Check sheet for the modelled part. Datum: model origin and axes. Units: mm. Face numbers are marked on the shaded views. A direction names the side the tool comes from. Round coordinates to 2 decimals unless told otherwise and drop trailing zeros. Order: outer loops, then holes, each group sorted by start corner. A loop starts at its lowest first (then second) coordinate and runs counter-clockwise, first axis right, second up.
(1) Sectioned sample at C-C, the plane x = 6.5. Enter the section's corners in (y, z).
(2) Sectioned sample at B-B, the plane z = 0. Enter the section's corners in (x, y).
(3) Sectioned sample at A-A, the plane y = -9.5. Enter the section's corners in (x, z), and give its area (3 significant figures).
(4) Sectioned sample at D-D, the plane y = -21. Enter the section's corners in (x, z).
(5) Tool access check on the marked faces 1 and 2. Record the directions out of +Z, -Z, +X, -X, +Y, -Y that give a thin tool (end or side, any length) a straight path to the whole face; none if there is none.
(6) Thickness scan on probe 1 along Z at (x, y) = (9.5, -20.5); probe 2 along X at (y, z) = (-9, -25); probe 3 along Z at (x, y) = (4, -12). Record the ranges inside material, lowest first.
```python
from build123d import *

# Parameters (mm, degrees)
BOSS_EXTRUDE1_DEPTH = 13
BOSS_EXTRUDE4_DEPTH = 2


with BuildPart() as part:
    # Sketch1 → Boss-Extrude1 (new body)
    with BuildSketch(Plane(origin=(0, 0, 0), x_dir=(0, 0, -1), z_dir=(1, 0, 0))):
        with BuildLine():
            Line((-50, 0), (-27.5, 0))
            ThreePointArc((-27.5, 0), (0, -27.5), (27.5, 0))
            Line((27.5, 0), (35, 0))
            Line((35, 0), (35, -35))
            Line((35, -35), (-50, -35))
            Line((-50, -35), (-50, 0))
        make_face()
    extrude(amount=BOSS_EXTRUDE1_DEPTH)

    # Sketch4 → Boss-Extrude4 (add)
    with BuildSketch(Plane(origin=(13, 0, 0), x_dir=(0, 0, -1), z_dir=(1, 0, 0))):
        with BuildLine():
            Line((35, 0), (35, -35))
            Line((35, -35), (-50, -35))
            Line((-50, -35), (-50, 0))
            Line((-50, 0), (-25.5, 0))
            ThreePointArc((-25.5, 0), (0, -25.5), (25.5, 0))
            Line((25.5, 0), (35, 0))
        make_face()
    extrude(amount=BOSS_EXTRUDE4_DEPTH)


solid = part.part
```
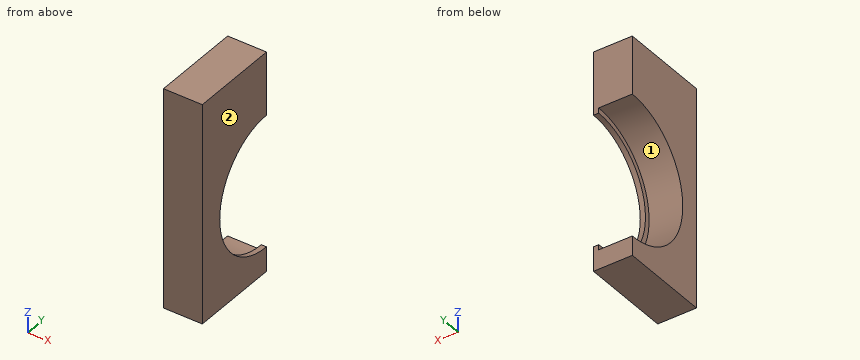
Derived:
1. outline: (-35, -35) - (0, -35) - (0, -27.5) arc R27.5 cw to (0, 27.5) - (0, 50) - (-35, 50) - close
2. outline: (0, -35) - (15, -35) - (15, -25.5) - (13, -25.5) - (13, -27.5) - (0, -27.5) - close
3. outline: (0, -35) - (15, -35) - (15, -23.66) - (13, -23.66) - (13, -25.81) - (0, -25.81) - close; (0, 25.81) - (13, 25.81) - (13, 23.66) - (15, 23.66) - (15, 50) - (0, 50) - close
3. area: 509 mm2
4. outline: (0, -35) - (15, -35) - (15, -14.47) - (13, -14.47) - (13, -17.76) - (0, -17.76) - close; (0, 17.76) - (13, 17.76) - (13, 14.47) - (15, 14.47) - (15, 50) - (0, 50) - close
5. face 1: -X, +Y
5. face 2: +Z, -Z, +X, +Y, -Y
6. probe 1: z = -35 to -18.33, 18.33 to 50
6. probe 2: x = 13 to 15
6. probe 3: z = -35 to -24.74, 24.74 to 50
